Design review of the part shown in the three views and the two pictorial views. Dimensions are in mm from the part's minimum x, y and z. A direction names the side the tool comes from. Round coordinates to 2 decimals unless told otherwise and drop trailing zeros. Loops run counter-clockwise (first coordinate to the right, second up) from the corner with the lowest first, then second, coordinate; pieces in that order, holes last. Notation, with made-up numbers: (13, 65.5) -> (26, 65.5) arc R19 ccw to (26, 74.5) -> close; hole circle Ø7 at (11.5, 69.25). An arc over 180 degrees is marked (long way). Use CSV: the item, a comma, the result in double quotes. Start each with the question number.
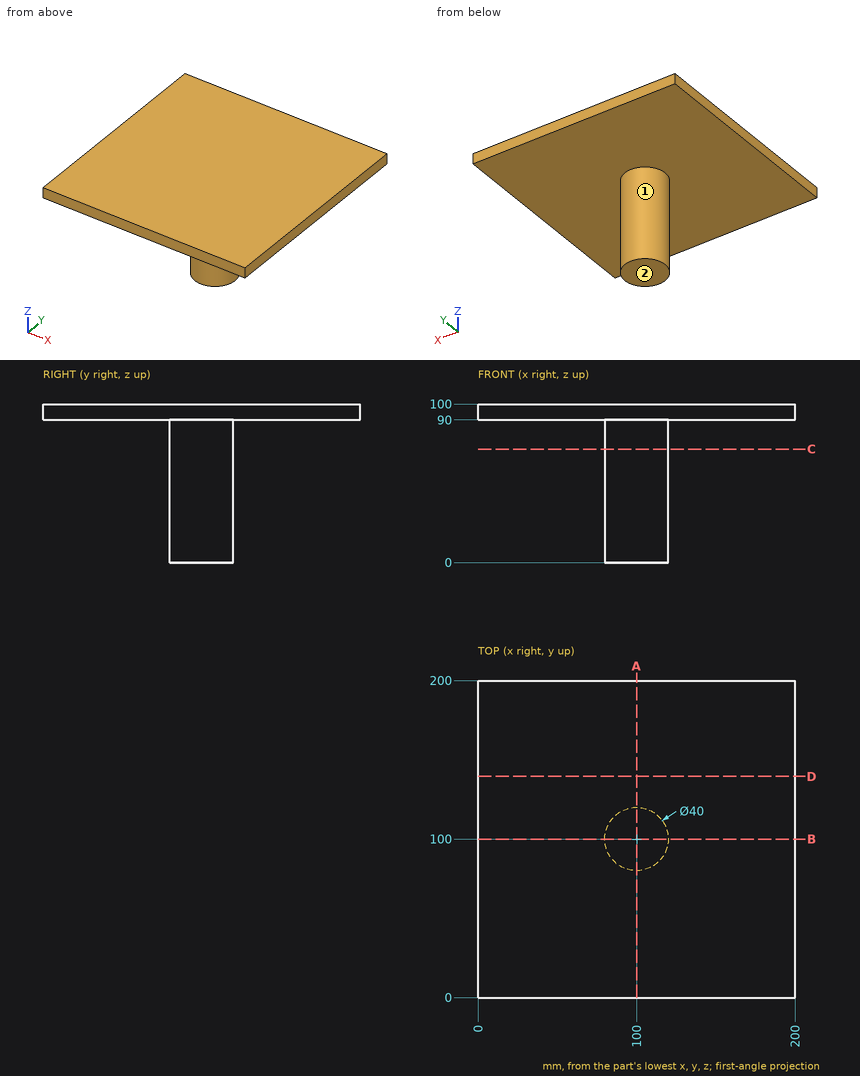
1. Take a section at C-C, the plane z = 71.5. Give the boundary of the cut face in (x, y), then the cut area to 3 significant figures.
2. Clearance check with flat-ended pins moving along their axes: P1, Ø1, axis at x = 104.5, z = 56.5, coming from the -Y side; P2, Ø10, axis at x = 158, y = 36, coming from the -Z side; P3, Ø2, axis at x = 78.5, z = 27.5, coming from the -Y side. State where each tip first meets the part, or that it passes through.
3. Take a section at D-D, the plane y = 139.5. Give the boundary of the cut face in (x, z), then the cut area to 3 significant figures.
4. For line 1 along Z through (x, y) = (76, 42.5); line 2 along X through (y, z) = (99.5, 62); line 3 along X through (y, z) = (104.5, 43), list the stretches that pass through material, from the lowest coordinate up. Write a range as from..to.
5. Take a section at A-A, the plane x = 100. Give the boundary of the cut face in (y, z), then the cut area to 3 significant figures.
6. For the marked faces 1 and 2, list the 3-axis set-ups (+Z, -Z, +X, -X, +Y, -Y) from which the entire face can be reached by the end or side of a thin tool; tool diameter is ignored.
Results:
1,outline,"circle Ø40 at (100, 100)"
1,area,"1,260 mm²"
2,P1,"y = 80.4"
2,P2,"z = 90"
2,P3,"through"
3,outline,"(0, 90) -> (200, 90) -> (200, 100) -> (0, 100) -> close"
3,area,"2,000 mm²"
4,line 1,"90..100"
4,line 2,"80.01..119.99"
4,line 3,"80.51..119.49"
5,outline,"(0, 90) -> (80, 90) -> (80, 0) -> (120, 0) -> (120, 90) -> (200, 90) -> (200, 100) -> (0, 100) -> close"
5,area,"5,600 mm²"
6,face 1,"-Z"
6,face 2,"-Z, +X, -X, +Y, -Y"
